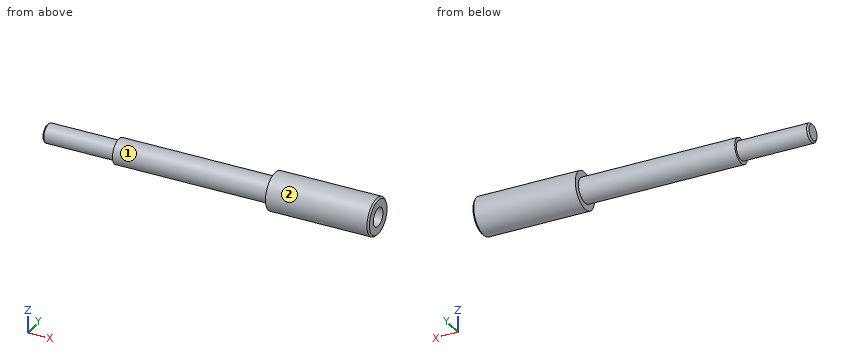
```python
from build123d import *


with BuildPart() as part:
    # Sketch_Shaft_Profile → Shaft_Revolve_12x33_8x50_M6x23_TappedM6x (revolve)
    with BuildSketch(Plane.XY, mode=Mode.PRIVATE) as shaft_revolve_12x33_8x50_m6x23_tappedm6x_sk:
        Polygon((0, 0), (0, 2.5), (0.5, 3), (23, 3), (23, 4), (73, 4), (73, 6), (105.5, 6), (106, 5.5), (106, 3), (92, 3), (92, 0), align=None)
    revolve(shaft_revolve_12x33_8x50_m6x23_tappedm6x_sk.sketch.rotate(Axis((-5, 0, 0), (1, 0, 0)), 90), axis=Axis((-5, 0, 0), (1, 0, 0)))


solid = part.part
```
CAD build for the part. Positions are in the model's coordinates, mm. Face numbers are marked on the shaded views. A direction names the side the tool comes from. Coordinates: 2 decimals unless noted, no trailing zeros. Order: outer loops, then holes, each group sorted by start corner. A loop starts at its lowest first (then second) coordinate and runs counter-clockwise, first axis right, second up. Notation, with made-up numbers: (62.5, 8.25) -> (102.5, 8.25) arc R22 ccw to (102.5, 28.25) -> close; hole circle Ø9 at (58, 4.25). An arc over 180 degrees is marked (long way). Use one line per item in the form item = value. Start each with the question number.
1) Band-saw the part on C-C on x = 83. Give the cut face in (y, z).
2) Band-saw the part on B-B on x = 99. Give the cut face in (y, z).
3) Drop flat-ended pins along their axis: pin 1 (6 mm diameter, centred on x = 48, z = -1, fed in from +Y); pin 2 (5 mm diameter, centred on x = 60, z = -3, fed in from -Y); pin 3 (3 mm diameter, centred on x = 93, z = 3.5, fed in from +Y). Give the stop position or say it passes through.
4) Band-saw the part on A-A on y = 0. Give the cut face in (x, z), then the cut area to 4 significant figures.
5) Drill centre lines: L1, parallel to Y at x = 100.5, z = 0; L2, parallel to X at y = 0.5, z = 5; L3, parallel to X at y = 3, z = -1.5. Where is each one in solid material? Low to high. Write a range as [from, to].
6) Band-saw the part on D-D on x = 21. Give the cut face in (y, z).
7) Tool access for the marked faces 1 and 2: list every direction of +Z, -Z, +X, -X, +Y, -Y with a clear straight run to the whole face (end or side of a thin tool).
Entries:
q1.outline = circle Ø12 at (0, 0)
q2.outline = circle Ø12 at (0, 0); hole circle Ø6 at (0, 0)
q3.pin_1 = 4
q3.pin_2 = -3.97
q3.pin_3 = 5.66
q4.outline = (0, -2.5) -> (0.5, -3) -> (23, -3) -> (23, -4) -> (73, -4) -> (73, -6) -> (105.5, -6) -> (106, -5.5) -> (106, -3) -> (92, -3) -> (92, 3) -> (106, 3) -> (106, 5.5) -> (105.5, 6) -> (73, 6) -> (73, 4) -> (23, 4) -> (23, 3) -> (0.5, 3) -> (0, 2.5) -> close
q4.area = 849.5 mm2
q5.L1 = [-6, -3], [3, 6]
q5.L2 = [73, 106]
q5.L3 = [23, 106]
q6.outline = circle Ø6 at (0, 0)
q7.face_1 = -X
q7.face_2 = +X, -X
